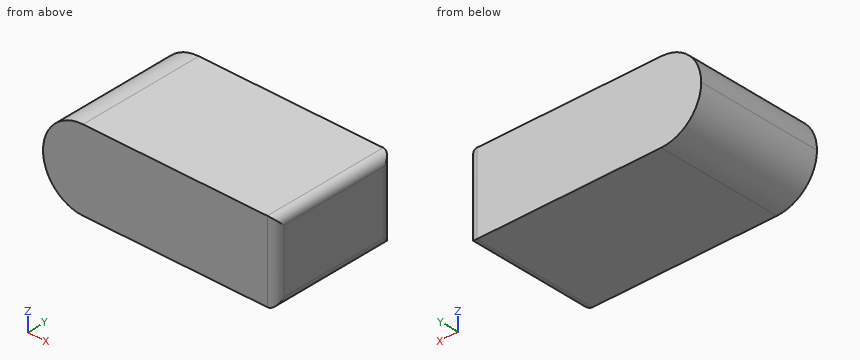
from build123d import *

# Parameters (mm, degrees)
F0_W     = 53.6
F0_H     = 29
F1_DEPTH = 18.4
F2_R     = 9.19999
F3_R     = 2


# Not quite as in the source:
# - a fillet or chamfer is up to 0.001 mm smaller than in the source, because OpenCascade refuses the exact size


with BuildPart() as f1:
    # F0 (on Top) → F1 (new body)
    with BuildSketch(Plane.XY):
        Rectangle(F0_W, F0_H)
    extrude(amount=F1_DEPTH)

    # F2 (radius 9.2 in the source; OpenCascade refuses exactly that, so slightly less here)
    f2_edges = [f1.edges().sort_by_distance(p)[0] for p in [
        (-26.8, 0, 18.4),
        (-26.8, 0, 0),
    ]]
    fillet(f2_edges, radius=F2_R)

    # F3
    f3_edges = [f1.edges().sort_by_distance(p)[0] for p in [
        (26.8, -14.5, 9.2),
        (26.8, 14.5, 9.2),
        (26.8, 0, 0),
        (26.8, 0, 18.4),
    ]]
    fillet(f3_edges, radius=F3_R)


solid = f1.part
Design review of the part built by this model. Coordinates are the model's own, in mm. Coordinates: 2 decimals unless noted, no trailing zeros. Order: outer loops, then holes, each group sorted by start corner. A loop starts at its lowest first (then second) coordinate and runs counter-clockwise, first axis right, second up.
Item 1: Take a section at C-C, the plane z = 15.75. Write out the cut boundary in (x, y), then the cut area to 3 significant figures.
Item 2: Take a section at B-B, the plane z = 13.5. Write out the cut boundary in (x, y).
Item 3: For pin 1 Ø4 at (y, z) = (8, 10) entering from -X; pin 2 Ø5 at (y, z) = (-0.5, 3.5) entering from -X, all flat-tipped, find the tip position at first contact; note any pin that passes through.
Item 4: For line 1 (X direction, y = -3.75, z = 7.25); line 2 (X direction, y = -11.25, z = 6.75), list the stretches that pass through material, from the lowest coordinate up.
The answers:
1. outline: (-24.06, -14.5) - (24.8, -14.5) arc R2 ccw to (26.8, -12.5) - (26.8, 12.5) arc R2 ccw to (24.8, 14.5) - (-24.06, 14.5) - close
1. area: 1,470 mm2
2. outline: (-25.73, -14.5) - (24.8, -14.5) arc R2 ccw to (26.8, -12.5) - (26.8, 12.5) arc R2 ccw to (24.8, 14.5) - (-25.73, 14.5) - close
3. pin 1: stops at x = -26.8
3. pin 2: stops at x = -26.23
4. line 1: x = -26.59 to 26.8
4. line 2: x = -26.47 to 26.8
